Source: CAD feature listing. Evaluate the final solid. Frame: model axes, mm. Face numbers are marked on the shaded views. A direction names the side the tool comes from. Round coordinates to 2 decimals unless told otherwise and drop trailing zeros. Order: outer loops, then holes, each group sorted by start corner. A loop starts at its lowest first (then second) coordinate and runs counter-clockwise, first axis right, second up. Notation, with made-up numbers: (33, 57.5) -> (56, 57.5) arc R11 ccw to (56, 69.5) -> close; hole circle Ø3 at (82, 23.25). An arc over 180 degrees is marked (long way). One line per item, written item: value. Start each with the question number.
1) Section A-A (y = 33). Return the cut outline in (x, z).
2) Reachability of the marked faces 1, 2, 3, 4 and 5 from +Z, -Z, +X, -X, +Y, -Y: full face, straight path, thin tool, end or side. Return the list, or none.
3) Ray query, L1, parallel to X at y = 25.5, z = 23; L2, parallel to Z at x = -17.5, y = 38; L3, parallel to Y at x = 48, z = 66. Return the intervals inside material, ascending.
4) Pin query (flat end, axial travel): P1, Ø7.5, axis at y = -23.5, z = 31, coming from the -X side; P2, Ø8, axis at y = -16.5, z = 52, coming from the -X side; P3, Ø5, axis at x = 54, y = 27.5, coming from the +Z side. Return the tip coordinate at first contact, or that it passes through.
5) Section B-B (z = -13). Return the cut outline in (x, y), and give its area (3 significant figures).
```python
from build123d import *

# Parameters (mm, degrees)
F1_DEPTH = 50
F0_W     = 30
F0_H     = 20
F2_DEPTH = 30
F4_DEPTH = 10


with BuildPart() as f1:
    # F0 (on Front) → F1 (new body, symmetric)
    with BuildSketch(Plane.XZ):
        Polygon((30, 20), (-75, 20), (-75, -20), (75, -20), (75, 20), (50, 20), align=None)
    extrude(amount=F1_DEPTH, both=True)

    # F0 (on Front) → F2 (join, symmetric)
    with BuildSketch(Plane.XZ):
        with BuildLine():
            Line((30, 35), (30, 20))
            Line((30, 20), (50, 20))
            Line((50, 20), (50, 35))
            ThreePointArc((50, 35), (54.3933982822, 45.6066017178), (65, 50))
            Line((65, 50), (85, 50))
            Line((85, 50), (85, 70))
            Line((85, 70), (65, 70))
            add(Edge.make_bspline(
                [(63.4724068362, 69.9666478108), (63.9831880061, 69.9787764937), (64.4924072773, 69.9898908886), (65, 70)],
                knots=[147.2868078235, 147.2868078235, 147.2868078235, 147.2868078235, 148.6606874732, 148.6606874732, 148.6606874732, 148.6606874732], degree=3))
            ThreePointArc((63.4724068362, 69.9666478108), (39.7169447976, 59.2026262962), (30, 35))
        make_face()
        with Locations((100, 60)):
            Rectangle(F0_W, F0_H)
    extrude(amount=F2_DEPTH, both=True)

    # F0 (on Front) → F3 (revolve)
    with BuildSketch(Plane.XZ):
        Polygon((115, 75), (115, 70), (115, 50), (115, 45), (145, 45), (145, 75), align=None)
    revolve(axis=Axis((115, 0, 60), (0, 0, 1)))

    # F0 (on Front) → F4 (join, symmetric)
    with BuildSketch(Plane.XZ):
        with BuildLine():
            add(Edge.make_bspline(
                [(-75, 20), (-63.9949885725, 55.7090067292), (8.7140966472, 68.6663920064), (63.4724068362, 69.9666478108)],
                knots=[0, 0, 0, 0, 147.2868078235, 147.2868078235, 147.2868078235, 147.2868078235], degree=3))
            Line((-75, 20), (30, 20))
            Line((30, 20), (30, 35))
            ThreePointArc((30, 35), (39.7169447976, 59.2026262962), (63.4724068362, 69.9666478108))
        make_face()
    extrude(amount=F4_DEPTH, both=True)


solid = f1.part
```
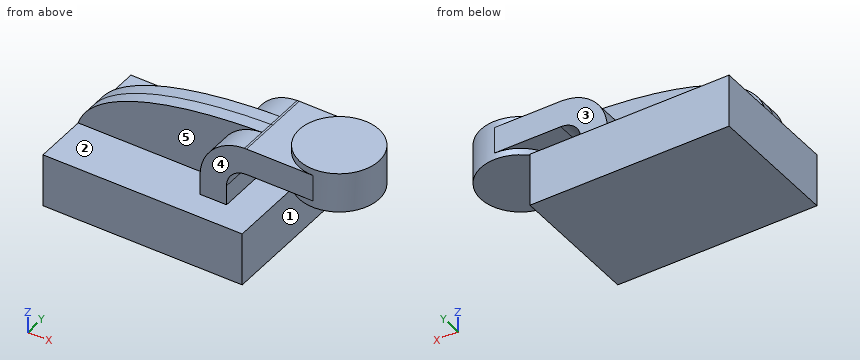
Findings:
1. outline: (-75, -20) -> (75, -20) -> (75, 20) -> (-75, 20) -> close
2. face 1: -Z, +X, +Y, -Y
2. face 2: none
2. face 3: +Z, +X, -X, +Y
2. face 4: +Z, +X, -X, -Y
2. face 5: +Z, -X, -Y
3. L1: 30 to 50
3. L2: -20 to 20
3. L3: -10 to 10
4. P1: x = 30
4. P2: x = 32.5
4. P3: z = 68.95
5. outline: (-75, -50) -> (75, -50) -> (75, 50) -> (-75, 50) -> close
5. area: 15,000 mm2
